Geometry check sheet. Reference: the model listing, model coordinates, mm. Face numbers are marked on the shaded views. A direction names the side the tool comes from. Round coordinates to 2 decimals unless told otherwise and drop trailing zeros. Order: outer loops, then holes, each group sorted by start corner. A loop starts at its lowest first (then second) coordinate and runs counter-clockwise, first axis right, second up.
(1) Set-up check for the marked faces 5 and 6: record each of +Z, -Z, +X, -X, +Y, -Y from which the full face is reachable in a straight line by a thin tool's end or side.
(2) Cross-section at B-B on x = -104. Enter the section's corners in (y, z).
(3) Draft check along Y on the marked faces 1, 2, 3 and 4. Enter one of: pulls with the +Y half, pulls with the -Y half, needs draft (parallel to the pull), parting line crosses it, or undercut.
(4) Cross-section at A-A on y = 6.5. Enter the section's corners in (x, z).
(5) Gauge pin test, flat ends, axial feed: P1, Ø10, axis at x = 92, y = -11.5, coming from the +Z side; P2, Ø12, axis at x = 36.5, z = 33.5, coming from the +Y side; P3, Ø5.5, axis at x = 115, y = -53.5, coming from the +Z side. Record the tip position at first contact, or that the pin passes through.
(6) Thickness scan on L1, parallel to Z at x = 57, y = -54 (3 decimals); L2, parallel to Y at x = -172, z = 51; L3, parallel to Z at x = -57, y = 61 (3 decimals). Record the ranges inside material, lowest first.
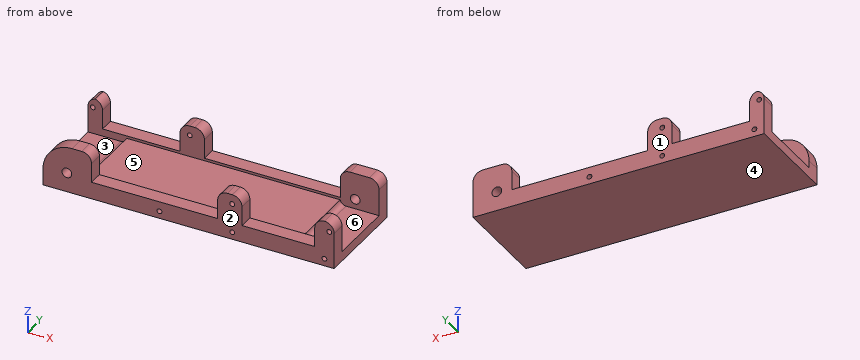
from build123d import *

# Parameters (mm, degrees)
F0_W         = 381
F0_H         = 127
F1_DEPTH     = 60.325
F2_W         = 88.9
F2_H         = 41.275
F3_DEPTH     = 381
F4_W         = 88.9
F4_H         = 6.35
F5_DEPTH     = 50.8
F6_T1_DEPTH  = 126.4671066227
F7_W         = 88.9
F7_H         = 6.35
F8_DEPTH     = 50.8
F9_T1_DEPTH  = 126.4671066227
F10_W        = 165.1
F10_H        = 37.973
F10_W_2      = 95.25
F11_DEPTH    = 19.05
F12_W        = 177.8
F12_H        = 37.973
F12_W_2      = 101.6
F13_DEPTH    = 19.05
F14_R        = 38.1
F15_R        = 12.69999
F16_T1_DEPTH = 82.55
F18_D        = 6.35
F18_DEPTH    = 12.7
F18_TIP      = 1.9077324654
F19_D        = 6.35
F19_DEPTH    = 25.4
F19_TIP      = 1.9077324654
F20_D        = 12.7
F20_DEPTH    = 25.4
F20_TIP      = 3.8154649308
F22_D        = 12.7
F22_DEPTH    = 25.4
F22_TIP      = 3.8154649308
F23_D        = 6.35
F23_DEPTH    = 12.7
F23_TIP      = 1.9077324654
F24_D        = 6.35
F24_DEPTH    = 25.4
F24_TIP      = 1.9077324654


# Not quite as in the source:
# - a fillet or chamfer that OpenCascade refuses, or shapes differently, is made with other operations: its cross-section is extruded or revolved along the edge and cut away or added
# - a fillet or chamfer is up to 0.001 mm smaller than in the source, because OpenCascade refuses the exact size


with BuildPart() as f1:
    # F0 (on Top) → F1 (new body)
    with BuildSketch(Plane.XY):
        Rectangle(F0_W, F0_H)
    extrude(amount=F1_DEPTH)

    # F2 (on face) → F3 (cut, through all)
    with BuildSketch(Plane.YZ.offset(190.5)):
        with Locations((0, 39.6875)):
            Rectangle(F2_W, F2_H)
    extrude(amount=-F3_DEPTH, mode=Mode.SUBTRACT)

    # F4 (on face) → F5 (cut)
    with BuildSketch(Plane.YZ.offset(190.5)):
        with Locations((0, 15.875)):
            Rectangle(F4_W, F4_H)
    extrude(amount=-F5_DEPTH, mode=Mode.SUBTRACT)

    # F6: fillet of radius 7.62 on 1 edges, made by hand

    # F6_s2 → F6_t1 (join)
    with BuildSketch(Plane.XZ.offset(-63.2335533113)):
        with BuildLine():
            ThreePointArc((139.7, 19.05), (142.2947324749, 14.5001288674), (147.2134213245, 12.7))
            Line((147.2134213245, 12.7), (139.7, 12.7))
            Line((139.7, 12.7), (139.7, 19.05))
        make_face()
    extrude(amount=F6_T1_DEPTH)

    # F7 (on face) → F8 (cut)
    with BuildSketch(Plane(origin=(-190.5, 0, 0), x_dir=(0, -1, 0), z_dir=(-1, 0, 0))):
        with Locations((0, 15.875)):
            Rectangle(F7_W, F7_H)
    extrude(amount=-F8_DEPTH, mode=Mode.SUBTRACT)

    # F9: fillet of radius 7.62 on 1 edges, made by hand

    # F9_s2 → F9_t1 (join)
    with BuildSketch(Plane.XZ.offset(-63.2335533113)):
        with BuildLine():
            ThreePointArc((-147.2134213245, 12.7), (-142.2947324749, 14.5001288674), (-139.7, 19.05))
            Line((-139.7, 19.05), (-139.7, 12.7))
            Line((-139.7, 12.7), (-147.2134213245, 12.7))
        make_face()
    extrude(amount=F9_T1_DEPTH)

    # F10 (on face) → F11 (cut, through all)
    with BuildSketch(Plane.XZ.offset(63.5)):
        with Locations((-44.45, 41.3385)):
            Rectangle(F10_W, F10_H)
        with Locations((117.475, 41.3385)):
            Rectangle(F10_W_2, F10_H)
    extrude(amount=-F11_DEPTH, mode=Mode.SUBTRACT)

    # F12 (on face) → F13 (cut, through all)
    with BuildSketch(Plane(origin=(0, 63.5, 0), x_dir=(-1, 0, 0), z_dir=(0, 1, 0))):
        with Locations((-50.8, 41.3385)):
            Rectangle(F12_W, F12_H)
        with Locations((120.65, 41.3385)):
            Rectangle(F12_W_2, F12_H)
    extrude(amount=-F13_DEPTH, mode=Mode.SUBTRACT)

    # F14
    f14_edges = [f1.edges().sort_by_distance(p)[0] for p in [
        (-190.5, -53.975, 60.325),
    ]]
    fillet(f14_edges, radius=F14_R)

    # F15 (radius 12.7 in the source; OpenCascade refuses exactly that, so slightly less here)
    f15_edges = [f1.edges().sort_by_distance(p)[0] for p in [
        (-127, -53.975, 60.325),
        (38.1, -53.975, 60.325),
        (69.85, -53.975, 60.325),
        (165.1, -53.975, 60.325),
        (190.5, -53.975, 60.325),
    ]]
    fillet(f15_edges, radius=F15_R)

    # F16: fillet of radius 12.7 on 6 edges, made by hand

    # F16_s2 → F16_t1 (cut)
    with BuildSketch(Plane.XZ.offset(-95.25)):
        with BuildLine():
            ThreePointArc((-184.15, 60.325), (-175.1697438789, 56.6052561211), (-171.45, 47.625))
            Line((-171.45, 47.625), (-171.45, 60.325))
            Line((-171.45, 60.325), (-184.15, 60.325))
        make_face()
        with BuildLine():
            ThreePointArc((-190.5, 47.625), (-186.7802561211, 56.6052561211), (-177.8, 60.325))
            Line((-177.8, 60.325), (-190.5, 60.325))
            Line((-190.5, 60.325), (-190.5, 47.625))
        make_face()
        with BuildLine():
            ThreePointArc((-57.15, 60.325), (-66.1302561211, 56.6052561211), (-69.85, 47.625))
            Line((-69.85, 47.625), (-69.85, 60.325))
            Line((-69.85, 60.325), (-57.15, 60.325))
        make_face()
        with BuildLine():
            ThreePointArc((-38.1, 47.625), (-41.8197438789, 56.6052561211), (-50.8, 60.325))
            Line((-50.8, 60.325), (-38.1, 60.325))
            Line((-38.1, 60.325), (-38.1, 47.625))
        make_face()
        with BuildLine():
            ThreePointArc((152.4, 60.325), (143.4197438789, 56.6052561211), (139.7, 47.625))
            Line((139.7, 47.625), (139.7, 60.325))
            Line((139.7, 60.325), (152.4, 60.325))
        make_face()
        with BuildLine():
            ThreePointArc((190.5, 47.625), (186.7802561211, 56.6052561211), (177.8, 60.325))
            Line((177.8, 60.325), (190.5, 60.325))
            Line((190.5, 60.325), (190.5, 47.625))
        make_face()
    extrude(amount=F16_T1_DEPTH, mode=Mode.SUBTRACT)

    # F18
    with Locations(Plane.XZ.offset(63.5)):
        with Locations((-38.1, 9.525), (57.15, 9.525), (177.8, 9.525)):
            Hole(F18_D / 2, depth=F18_DEPTH)
            with Locations((0, 0, -(F18_DEPTH + F18_TIP / 2))):  # 118° drill point
                Cone(0, F18_D / 2, F18_TIP, mode=Mode.SUBTRACT)

    # F19
    with Locations(Plane.XZ.offset(63.5)):
        with Locations((57.15, 47.752), (184.15, 47.752)):
            Hole(F19_D / 2, depth=F19_DEPTH)
            with Locations((0, 0, -(F19_DEPTH + F19_TIP / 2))):  # 118° drill point
                Cone(0, F19_D / 2, F19_TIP, mode=Mode.SUBTRACT)

    # F20
    with Locations(Plane.XZ.offset(63.5)):
        with Locations((-159.258, 25.4)):
            Hole(F20_D / 2, depth=F20_DEPTH)
            with Locations((0, 0, -(F20_DEPTH + F20_TIP / 2))):  # 118° drill point
                Cone(0, F20_D / 2, F20_TIP, mode=Mode.SUBTRACT)

    # F22
    with Locations(Plane(origin=(0, 63.5, 0), x_dir=(-1, 0, 0), z_dir=(0, 1, 0))):
        with Locations((-159.258, 25.4)):
            Hole(F22_D / 2, depth=F22_DEPTH)
            with Locations((0, 0, -(F22_DEPTH + F22_TIP / 2))):  # 118° drill point
                Cone(0, F22_D / 2, F22_TIP, mode=Mode.SUBTRACT)

    # F23
    with Locations(Plane(origin=(0, 63.5, 0), x_dir=(-1, 0, 0), z_dir=(0, 1, 0))):
        with Locations((-38.1, 9.652), (57.15, 9.652), (177.8, 9.652)):
            Hole(F23_D / 2, depth=F23_DEPTH)
            with Locations((0, 0, -(F23_DEPTH + F23_TIP / 2))):  # 118° drill point
                Cone(0, F23_D / 2, F23_TIP, mode=Mode.SUBTRACT)

    # F24
    with Locations(Plane(origin=(0, 63.5, 0), x_dir=(-1, 0, 0), z_dir=(0, 1, 0))):
        with Locations((57.15, 47.752), (184.15, 47.752)):
            Hole(F24_D / 2, depth=F24_DEPTH)
            with Locations((0, 0, -(F24_DEPTH + F24_TIP / 2))):  # 118° drill point
                Cone(0, F24_D / 2, F24_TIP, mode=Mode.SUBTRACT)


solid = f1.part
Found:
1. face 5: +Z, +X, -X
1. face 6: +Z, +X
2. outline: (-63.5, 0) - (63.5, 0) - (63.5, 22.35) - (44.45, 22.35) - (44.45, 19.05) - (-44.45, 19.05) - (-44.45, 22.35) - (-63.5, 22.35) - close
3. face 1: pulls with the +Y half
3. face 2: pulls with the -Y half
3. face 3: undercut
3. face 4: needs draft
4. outline: (-190.5, 0) - (190.5, 0) - (190.5, 12.7) - (147.21, 12.7) arc R7.62 cw to (139.7, 19.05) - (-139.7, 19.05) arc R7.62 cw to (-147.21, 12.7) - (-190.5, 12.7) - close
5. P1: stops at z = 19.05
5. P2: stops at y = -44.45
5. P3: stops at z = 22.35
6. L1: z = 0 to 6.354, 12.696 to 44.581, 50.923 to 60.325
6. L2: y = -63.5 to -44.45, 44.45 to 63.5
6. L3: z = 0 to 6.481, 12.823 to 44.581, 50.923 to 60.325
